Read the model definition and answer for the solid it produces. Units are mm, in the model's axes. A direction names the side the tool comes from. Coordinates: 2 decimals unless noted, no trailing zeros. Loops run counter-clockwise (first coordinate to the right, second up) from the corner with the lowest first, then second, coordinate; pieces in that order, holes last.
Q1. Section A-A (y = -18.5) is taken. Give the vertices of the cut face in (x, z).
Q2. Flat-ended cylindrical pins translate along their axes: P1, Ø5, axis at x = 131, z = 314, coming from the +Y side; P2, Ø3, axis at x = 4, z = 104.5, coming from the -Y side; P3, Ø1.5, axis at x = 142, z = 120.5, coming from the -Y side. Find the tip coordinate at first contact, or state that the pin passes through.
Q3. The mould has two halves that part along X. Classify faces 3 (the face through (33, 3, -475)), 4 (the face through (-145, -29, -7)), 5 (the face through (140, -28, 7)): pulls with the +X half, pulls with the -X half, needs draft (parallel to the pull), parting line crosses it, or undercut.
Q4. Which of the six approach directions +Z, -Z, +X, -X, +Y, -Y give full straight-line access (tool end or side, diameter ignored) to faces 1 (the face through (-140, -28, -7)), 2 (the face through (33, 3, 475))?
Q5. Section C-C (z = 106.5) is taken. Give the vertices of the cut face in (x, y).
Q6. Straight lines are drawn through the part: line 1 (Z direction, x = 110, y = 4); line 2 (X direction, y = -28, z = 431.5); line 3 (Z direction, x = 0, y = 2). For each, find the intervals that lie inside material, in ascending order.
Q7. Section B-B (z = 0) is taken. Give the vertices of the cut face in (x, y).
Q8. Section D-D (y = -70) is taken. Give the vertices of the cut face in (x, z), then the cut area to 3 significant figures.
Autodesk Inventor part; units mm, degrees
ref_plane "Arbeitsebene1" through (0, 0, 0) normal (1, 0, 0) x (0, 1, 0)
ref_plane "XZ Plane" through (0, 0, 0) normal (0, 1, 0) x (-1, 0, 0)
ref_plane "XY Plane" through (0, 0, 0) normal (0, 0, 1) x (1, 0, 0)
sketch "Skizze1" plane through (0, 0, 0) normal (0, 1, 0) x (-1, 0, 0)
  line L0 (-140, 475) -> (140, 475)
  line L1 (140, 475) -> (140, -475)
  line L2 (140, -475) -> (-140, -475)
  line L3 (-140, -475) -> (-140, 475)
  line L4 (-140, 475) -> (140, -475) construction
  line L5 (140, 475) -> (-140, -475) construction
  point P0 (0, 0)
  dimension "d0" = 950
  dimension "d1" = 280
extrude "Grobblech4" add sketch "Skizze1" along normal blind 5
sketch "Skizze2" plane through (140, 0, 475) normal (1, 0, 0) x (0, 1, 0)
  line L0 (0, -950) -> (0, 0)
  line L1 (0, 0) -> (-91, 0)
  line L2 (-91, 0) -> (-91, -950)
  line L3 (-91, -950) -> (0, -950)
edge flange "Lasche1" height 96 angle 90 thickness 5 bend radius 5 thickness toward (1, 0, 0) relief tear relief width 5 relief depth 2.5 corner gap 5 corner form 0 edges at (140, 0, 0) (-140, 0, 0) wall of the first edge with corners at (140, 0, -475) (140, 0, 475) (140, -91, 475) (140, -91, -475)
bend "Biegung1"
corner "Ecke1"
sketch "Skizze3" plane through (145, -92.952, 475) normal (1, 0, 0) x (0, 0, -1)
  line L0 (0, 56) -> (10, 1.952)
  line L1 (74, 1.952) -> (84, 56)
  line L2 (84, 56) -> (866, 56)
  line L3 (866, 56) -> (876, 1.952)
  line L4 (876, 1.952) -> (940, 1.952)
  line L5 (940, 1.952) -> (950, 56)
  line L6 (10, 1.952) -> (74, 1.952)
  line L7 (950, 87.952) -> (0, 87.952)
  line L8 (0, 1.952) -> (0, 87.952)
  line L9 (950, 1.952) -> (0, 1.952)
  line L10 (950, 87.952) -> (950, 1.952)
  line L11 (950, 1.952) -> (0, 1.952)
  point P0 (475, 92.952)
  point P1 (42, 1.952)
  point P2 (908, 1.952)
  point P3 (950, 56)
  point P4 (940, 1.952)
  point P5 (74, 1.952)
  point P6 (876, 1.952)
  point P7 (10, 1.952)
  point P8 (0, 56)
  dimension "d15" = 10
  dimension "d16" = 64
  dimension "d17" = 10
  dimension "d18" = 10
  dimension "d19" = 64
  dimension "d22" = 54.048
extrude "Extrusion2" cut sketch "Skizze3" against normal up to surface (5 mm away) contours L0 L9 L8 | L1 L2 L3 L9 | L10 L9 L5
ref_plane "Arbeitsebene1" through (0, 0, 0) normal (1, 0, 0) x (0, 1, 0)
mirror "Spiegeln1" about plane through (0, 0, 0) normal (1, 0, 0) of "Extrusion2"
sketch "Skizze4" plane through (0, 5, 0) normal (0, 1, 0) x (1, 0, 0)
  line L0 (-135, 475) -> (135, 475)
  point P0 (110, 391)
  point P1 (-110, 391)
  point P2 (0, 0)
  dimension "d34" = 220
  dimension "d76" = 84
  dimension "d77" = 110
hole "Bohrung1" at (110, 5, -391) at (-110, 5, -391) direction (0, -1, 0) diameter 12 depth 5
sketch "Skizze5" plane through (0, 5, 0) normal (0, 1, 0) x (1, 0, 0)
  circle A0 centre (-110, 391) radius 6
  point P0 (110, 271)
  point P1 (-110, 271)
  point P2 (110, 391)
  point P3 (0, 0)
  dimension "d43" = 120
hole "Bohrung2" at (110, 5, -271) at (-110, 5, -271) direction (0, -1, 0) diameter 12 end through all
sketch "Skizze6" plane through (0, 5, 0) normal (0, 1, 0) x (1, 0, 0)
  circle A0 centre (110, 271) radius 6
  point P0 (122.5, 176)
  point P1 (-122.5, 176)
  point P2 (0, 0)
  dimension "d55" = 245
  dimension "d88" = 122.5
  dimension "d89" = 95
hole "Bohrung3" at (122.5, 5, -176) at (-122.5, 5, -176) direction (0, -1, 0) diameter 10.106 end through all
sketch "Skizze7" plane through (0, 5, 0) normal (0, 1, 0) x (1, 0, 0)
  line L0 (145, 475) -> (145, -475)
  line L1 (0, 0) -> (0, -582.3396) construction
  point P0 (131, -314)
  point P1 (-124, -314)
  dimension "d73" = 255
  dimension "d79" = 14
  dimension "d80" = 314
hole "Bohrung5" at (131, 5, 314) at (-124, 5, 314) direction (0, -1, 0) diameter 8.376 depth 5
sketch "Skizze8" plane through (0, 5, 0) normal (0, 1, 0) x (1, 0, 0)
  point P0 (0, 0)
  point P1 (0, 0)
hole "Bohrung6" at (0, 5, 0) direction (0, -1, 0) diameter 20 depth 5
equation "\"d31\" = Stärke"
equation "\"d64\" = d72"
equation "\"d82\" = d72"
equation "\"d2\" = Stärke"
equation "\"d3\" = BreiteBiegungsfreistellung"
equation "\"d4\" = TiefeBiegungsfreistellung"
equation "\"d5\" = MinimalRest"
equation "\"d6\" = Übergangsradius"
equation "\"d9\" = Biegeradius"
equation "\"d10\" = GrößeEckenfreistellung"
equation "\"d11\" = Abstandsgröße"
equation "\"d12\" = JacobiRadiusGröße"
equation "\"Biegeradius\" = Stärke"
equation "\"BreiteBiegungsfreistellung\" = Stärke"
equation "\"TiefeBiegungsfreistellung\" = 0.5 * Stärke"
equation "\"Übergangsradius\" = Biegeradius"
equation "\"JacobiRadiusGröße\" = Biegeradius"
equation "\"Abstandsgröße\" = Stärke"
properties part number "9" material "Aluminium 6061"
Numbers:
1. outline: (-145, -475) - (-140, -475) - (-140, 475) - (-145, 475) - close; (140, -475) - (145, -475) - (145, 475) - (140, 475) - close
2. P1: passes through
2. P2: stops at y = 0
2. P3: stops at y = -36.95
3. face 3: needs draft
3. face 4: pulls with the -X half
3. face 5: undercut
4. face 1: +Z, -Z, -Y
4. face 2: +Z, +X, -X, +Y, -Y
5. outline: (-145, -36.95) - (-140, -36.95) - (-140, -5) arc R5 cw to (-135, 0) - (135, 0) arc R5 cw to (140, -5) - (140, -36.95) - (145, -36.95) - (145, -5) arc R10 ccw to (135, 5) - (-135, 5) arc R10 ccw to (-145, -5) - close
6. line 1: z = -475 to -397, -385 to -277, -265 to 475
6. line 2: x = -145 to -140, 140 to 145
6. line 3: z = -475 to -10, 10 to 475
7. outline: (-145, -36.95) - (-140, -36.95) - (-140, -5) arc R5 cw to (-135, 0) - (-10, 0) - (-10, 5) - (-135, 5) arc R10 ccw to (-145, -5) - close; (10, 0) - (135, 0) arc R5 cw to (140, -5) - (140, -36.95) - (145, -36.95) - (145, -5) arc R10 ccw to (135, 5) - (10, 5) - close
8. outline: (-145, -468.89) - (-140, -468.89) - (-140, -397.11) - (-145, -397.11) - close; (-145, 397.11) - (-140, 397.11) - (-140, 468.89) - (-145, 468.89) - close; (140, -468.89) - (145, -468.89) - (145, -397.11) - (140, -397.11) - close; (140, 397.11) - (145, 397.11) - (145, 468.89) - (140, 468.89) - close
8. area: 1,440 mm2
